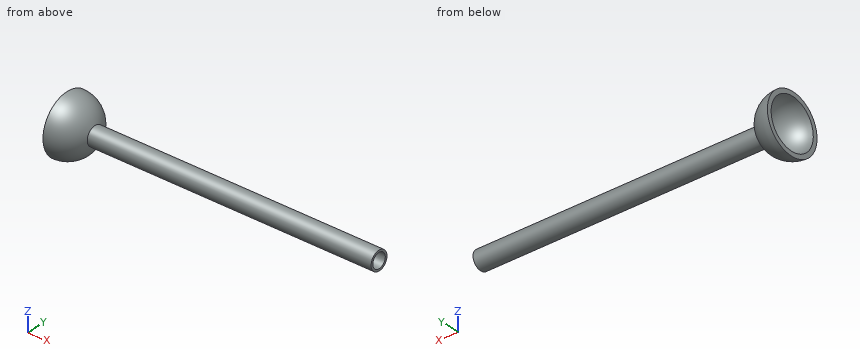
```python
from build123d import *


with BuildPart() as part:
    # Sketch1 → Revolve1 (revolve)
    with BuildSketch(Plane(origin=(0, 0, 0), x_dir=(1, 0, 0), z_dir=(0, 1, 0))):
        with BuildLine():
            Line((0, 12.7), (0, 10.795))
            ThreePointArc((0, 10.795), (7.633217703, 7.633217703), (10.795, 0))
            Line((10.795, 0), (12.7, 0))
            ThreePointArc((12.7, 0), (12.597580707, 1.609646024), (12.291974752, 3.193330031))
            Line((12.291974752, 3.193330031), (136.525, 3.193330031))
            Line((136.525, 3.193330031), (136.525, 4.074251535))
            Line((136.525, 4.074251535), (12.028735363, 4.074251535))
            ThreePointArc((12.028735363, 4.074251535), (7.400912292, 10.320682983), (0, 12.7))
        make_face()
    revolve(axis=Axis((0, 0, 0), (1, 0, 0)))


solid = part.part
```
Geometry check sheet. Reference: the model listing, model coordinates, mm. Round coordinates to 2 decimals unless told otherwise and drop trailing zeros. Loops run counter-clockwise (first coordinate to the right, second up) from the corner with the lowest first, then second, coordinate; pieces in that order, holes last. Notation, with made-up numbers: M 70.5,81.5 L 100.5,81.5 A20 ccw 100.5,100.5 Z; hole C -8.5,-26 d7. An arc over 180 degrees is marked long. Return JSON: item names as keys, results as strings. Group by question number.
(1) Scan lines: line 1 along Y through (x, z) = (40, -0.25); line 2 along Z through (x, y) = (71, -2.5); line 3 along X through (y, z) = (-5.5, -7.5). Record each from-to range of solid material in increasing order. Write a range as [from, to].
(2) Section check A-A, the plane z = 0. Enter the section's corners in (x, y) (3 decimals).
(3) Section check C-C, the plane x = 80. Enter the section's corners in (y, z).
(4) Section check D-D, the plane z = 9.5. Enter the section's corners in (x, y).
(5) Go/stop test with flat-tipped pins: pin 1 (12 mm diameter, centred on x = 40, y = 3, fed in from +Z); pin 2 (12 mm diameter, centred on x = 80.5, y = -8.5, fed in from -Z); pin 3 (5 mm diameter, centred on x = 108.5, z = -1, fed in from +Y); pin 4 (1.5 mm diameter, centred on x = 45, y = -5.5, fed in from +Z). Record where each tip stops, or that it passes through.
Data:
{
 "1": {"line 1": "[-4.07, -3.18], [3.18, 4.07]", "line 2": "[-3.22, -1.99], [1.99, 3.22]", "line 3": "[5.48, 8.65]"},
 "2": {"outline": "M 0,-12.7 A12.7 ccw 12.029,-4.074 L 136.525,-4.074 L 136.525,-3.193 L 12.292,-3.193 A12.7 ccw 12.292,3.193 L 136.525,3.193 L 136.525,4.074 L 12.029,4.074 A12.7 ccw 0,12.7 L 0,10.795 A10.795 cw 0,-10.795 Z"},
 "3": {"outline": "C 0,0 d8.15; hole C 0,0 d6.39"},
 "4": {"outline": "M 0,-8.43 A8.43 ccw 0,8.43 L 0,5.13 A5.13 cw 0,-5.13 Z"},
 "5": {"pin 1": "z = 4.07", "pin 2": "z = -3.22", "pin 3": "y = 4.07", "pin 4": "through"}
}
